Verification items for the finished model (mm, model axes). A direction names the side the tool comes from. Round coordinates to 2 decimals unless told otherwise and drop trailing zeros. Order: outer loops, then holes, each group sorted by start corner. A loop starts at its lowest first (then second) coordinate and runs counter-clockwise, first axis right, second up.
```python
from build123d import *

# Parameters (mm, degrees)
ESQUISSE1_W             = 419
ESQUISSE1_H             = 134
BOSS_EXTRU_1_DEPTH      = 22
ESQUISSE3_W             = 419
ESQUISSE3_H             = 134
ESQUISSE3_W_2           = 375
ESQUISSE3_H_2           = 90
BOSS_EXTRU_2_DEPTH      = 55
ESQUISSE4_R             = 28
ENL_V_MAT_EXTRU_1_DEPTH = 3


with BuildPart() as part:
    # Esquisse1 → Boss.-Extru.1 (new body)
    with BuildSketch(Plane.XY):
        with Locations((209.5, -67)):
            Rectangle(ESQUISSE1_W, ESQUISSE1_H)
    extrude(amount=BOSS_EXTRU_1_DEPTH)

    # Esquisse3 → Boss.-Extru.2 (add)
    with BuildSketch(Plane.XY.offset(22)):
        with Locations((209.5, -67)):
            Rectangle(ESQUISSE3_W, ESQUISSE3_H)
        with Locations((209.5, -67)):
            Rectangle(ESQUISSE3_W_2, ESQUISSE3_H_2, mode=Mode.SUBTRACT)
    extrude(amount=BOSS_EXTRU_2_DEPTH)

    # Esquisse4 → Enlèv. mat.-Extru.1 (cut)
    with BuildSketch(Plane.XY.offset(22)):
        with Locations((59, -67)):
            Circle(ESQUISSE4_R)
        with Locations((134, -67)):
            Circle(ESQUISSE4_R)
        with Locations((209, -67)):
            Circle(ESQUISSE4_R)
        with Locations((284, -67)):
            Circle(ESQUISSE4_R)
        with Locations((359, -67)):
            Circle(ESQUISSE4_R)
    extrude(amount=-ENL_V_MAT_EXTRU_1_DEPTH, mode=Mode.SUBTRACT)


solid = part.part
```
1) Sectioned sample at D-D on y = -28. Record the cut outline in (x, z), then the cut area to 3 significant figures.
2) Sectioned sample at C-C on x = 59. Record the cut outline in (y, z), then the cut area to 3 significant figures.
3) Tool access check on faces 1 (the flat face through (160, -21, 77)), 2 (the cylindrical face through (234.865, -77.724, 20.521)). Record the directions out of +Z, -Z, +X, -X, +Y, -Y that give a thin tool (end or side, any length) a straight path to the whole face; none if there is none.
4) Sectioned sample at A-A on z = 48.5. Record the cut outline in (x, y).
5) Draft check along X on faces 3 (the flat face through (59, -67, 19)), 4 (the flat face through (0, -68, 38)), 5 (the flat face through (207, -134, 38)). Enter one of: released by +X, released by -X, zero draft, split by the parting line, or undercut.
6) Sectioned sample at B-B on y = -67. Record the cut outline in (x, z).
7) Scan lines: probe 1 along Y at (x, z) = (362.5, 58); probe 2 along X at (y, z) = (-26, 45); probe 3 along Z at (x, y) = (157, -63). Record each from-to range of solid material in increasing order.
8) Go/stop test with a flat-tipped pin: pin 1 Ø17 at (x, y) = (359, -61.5) entering from +Z. Record where the tip stops, or that it passes through.
Returned:
1. outline: (0, 0) - (419, 0) - (419, 77) - (397, 77) - (397, 22) - (22, 22) - (22, 77) - (0, 77) - close
1. area: 11,600 mm2
2. outline: (-134, 0) - (0, 0) - (0, 77) - (-22, 77) - (-22, 22) - (-39, 22) - (-39, 19) - (-95, 19) - (-95, 22) - (-112, 22) - (-112, 77) - (-134, 77) - close
2. area: 5,200 mm2
3. face 1: +Z, +X, -X, +Y, -Y
3. face 2: +Z
4. outline: (0, -134) - (419, -134) - (419, 0) - (0, 0) - close; hole (22, -112) - (397, -112) - (397, -22) - (22, -22) - close
5. face 3: undercut
5. face 4: released by -X
5. face 5: zero draft
6. outline: (0, 0) - (419, 0) - (419, 77) - (397, 77) - (397, 22) - (387, 22) - (387, 19) - (331, 19) - (331, 22) - (312, 22) - (312, 19) - (256, 19) - (256, 22) - (237, 22) - (237, 19) - (181, 19) - (181, 22) - (162, 22) - (162, 19) - (106, 19) - (106, 22) - (87, 22) - (87, 19) - (31, 19) - (31, 22) - (22, 22) - (22, 77) - (0, 77) - close
7. probe 1: y = -134 to -112, -22 to 0
7. probe 2: x = 0 to 22, 397 to 419
7. probe 3: z = 0 to 19
8. pin 1: stops at z = 19
